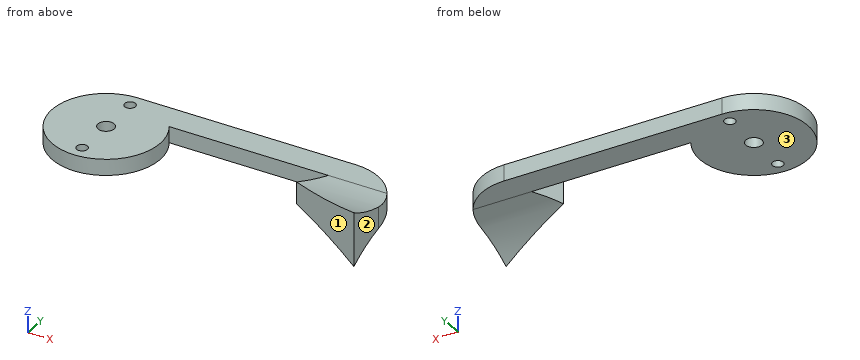
from build123d import *

# Parameters (mm, degrees)
SKETCH1_R           = 1.5
BOSS_EXTRUDE1_DEPTH = 1.5
BOSS_EXTRUDE2_DEPTH = 5
CUT_EXTRUDE1_START  = -12.113249
SKETCH3_OUTSIDE_W   = 24.806
SKETCH3_OUTSIDE_H   = 34.806
CUT_EXTRUDE1_DEPTH  = 15
SKETCH4_R           = 1
CUT_EXTRUDE2_DEPTH  = 52.402821


with BuildPart() as part:
    # Sketch1 → Boss-Extrude1 (new, symmetric)
    with BuildSketch(Plane.XY):
        with BuildLine():
            Line((0, 10), (40, 10))
            ThreePointArc((40, 10), (47.071068, 7.071068), (50, 0))
            Line((50, 0), (35, 0))
            Line((35, 0), (37.886751, 5))
            Line((37.886751, 5), (8.660254, 5))
            ThreePointArc((8.660254, 5), (-5, -8.660254), (0, 10))
        make_face()
        Circle(SKETCH1_R, mode=Mode.SUBTRACT)
    extrude(amount=BOSS_EXTRUDE1_DEPTH, both=True)

    # Sketch2 → Boss-Extrude2 (add, symmetric)
    with BuildSketch(Plane.XY):
        with BuildLine():
            Line((37.886751, 5), (37.886751, 10))
            Line((37.886751, 10), (40, 10))
            ThreePointArc((40, 10), (47.071068, 7.071068), (50, 0))
            Line((50, 0), (50, -7.642882))
            Line((50, -7.642882), (35, 0))
            Line((35, 0), (37.886751, 5))
        make_face()
    extrude(amount=BOSS_EXTRUDE2_DEPTH, both=True)

    # Sketch3 outside → Cut-Extrude1 (cut)
    with BuildSketch(Plane.ZY.offset(-37.886751).offset(CUT_EXTRUDE1_START)):
        Rectangle(SKETCH3_OUTSIDE_W, SKETCH3_OUTSIDE_H)
        with BuildLine():
            Line((-1.5, 10), (-1.5, 5))
            ThreePointArc((-1.5, 5), (-2.391151, -1.559201), (-5, -7.642882))
            Line((-5, -7.642882), (5, -7.642882))
            ThreePointArc((5, -7.642882), (2.391151, -1.559201), (1.5, 5))
            Line((1.5, 5), (1.5, 10))
            Line((1.5, 10), (-1.5, 10))
        make_face(mode=Mode.SUBTRACT)
    extrude(amount=CUT_EXTRUDE1_DEPTH, mode=Mode.SUBTRACT)

    # Sketch4 → Cut-Extrude2 (cut, through all)
    with BuildSketch(Plane(origin=(0, 0, -1.5), x_dir=(-1, 0, 0), z_dir=(0, 0, -1))):
        with Locations((0, 7.5)):
            Circle(SKETCH4_R)
        with Locations((0, -7.5)):
            Circle(SKETCH4_R)
    extrude(amount=-CUT_EXTRUDE2_DEPTH, mode=Mode.SUBTRACT)


solid = part.part
The listing builds one solid part. Answer for the finished solid, in the listing's coordinates (mm). Face numbers are marked on the shaded views. Give positions to 0.01 mm unless a question says otherwise; leave off trailing zeros. Order: outer loops, then holes, each group sorted by start corner. A loop starts at its lowest first (then second) coordinate and runs counter-clockwise, first axis right, second up. Notation, with made-up numbers: (13.25, 50) - (41.25, 50) arc R15 cw to (41.25, 60) - close; hole circle Ø5 at (53, 73). An arc over 180 degrees is marked (long way). Use one line per item in the form item = value.
1) Find section A-A on z = 0. Determine the outline of the cut face in (x, y).
Verdict:
outline = (0, 10) arc R10 ccw (long way) to (8.66, 5) - (37.89, 5) - (35, 0) - (50, -7.64) - (50, 0) arc R10 ccw to (40, 10) - close; hole circle Ø3 at (0, 0); hole circle Ø2 at (0, -7.5); hole circle Ø2 at (0, 7.5)
2) Consider probe 1 along Y at (x, z) = (0, -0.65); probe 2 along Y at (x, z) = (19.5, 0.5); probe 3 along Z at (x, y) = (2, -8.25). Determine where each line is inside the solid, lowest interval first. Write a range as [from, to].
Verdict:
probe_1 = [-10, -8.5], [-6.5, -1.5], [1.5, 6.5], [8.5, 10]
probe_2 = [5, 10]
probe_3 = [-1.5, 1.5]
3) Each of these flat-tipped pins is pushed along its axis until it touches: pin 1 (2 mm diameter, centred on x = 16.5, y = 4.5, fed in from +Z); pin 2 (2.5 mm diameter, centred on x = 17, z = -0.5, fed in from -Y); pin 3 (4 mm diameter, centred on y = 5, z = -2.5, fed in from -X). Where does it stop, or does it pass through?
Verdict:
pin_1 = 1.5
pin_2 = 5
pin_3 = -9.45
4) Find section C-C on x = 18. Determine the outline of the cut face in (y, z), and give its area (3 significant figures).
Verdict:
outline = (5, -1.5) - (10, -1.5) - (10, 1.5) - (5, 1.5) - close
area = 15.0 mm^2
5) The mould has two halves that part along X. Classify the marked faces 1, 2 and 3: released by +X, released by -X, zero draft, split by the parting line, or undercut.
Verdict:
face_1 = undercut
face_2 = released by +X
face_3 = zero draft
6) Find section B-B on y = 7.5. Determine the outline of the cut face in (x, z).
Verdict:
outline = (-6.61, -1.5) - (-1, -1.5) - (-1, 1.5) - (-6.61, 1.5) - close; (1, -1.5) - (46.61, -1.5) - (46.61, 1.5) - (1, 1.5) - close
7) Find section D-D on y = 3.25. Determine the outline of the cut face in (x, z).
Verdict:
outline = (-9.46, -1.5) - (9.46, -1.5) - (9.46, 1.5) - (-9.46, 1.5) - close; (36.88, -1.56) - (49.46, -1.56) - (49.46, 1.56) - (36.88, 1.56) - close
